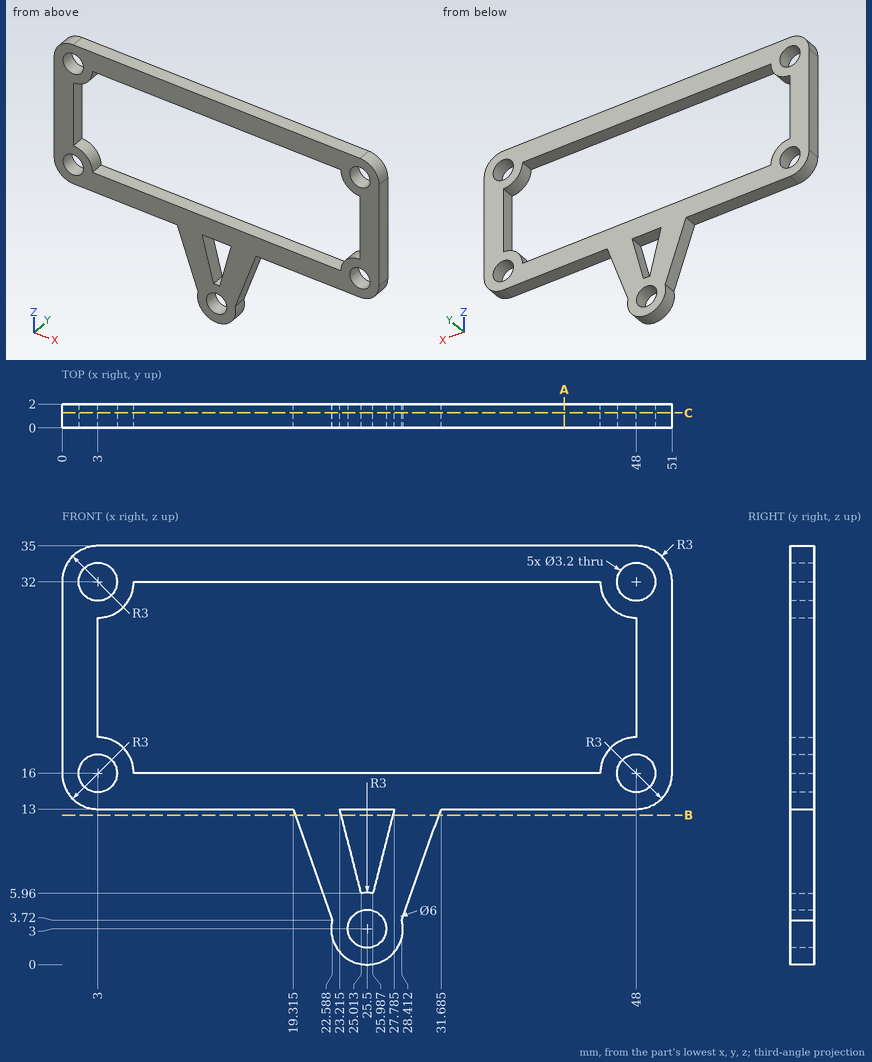
Geometry check sheet. Reference: drawing and pictorial views, mm from the part's lowest x, y, z. Coordinates: 2 decimals unless noted, no trailing zeros. Order: outer loops, then holes, each group sorted by start corner. A loop starts at its lowest first (then second) coordinate and runs counter-clockwise, first axis right, second up. Notation, with made-up numbers: (-18.5, 43.5) -> (10.5, 43.5) arc R16 ccw to (10.5, 70.5) -> close; hole circle Ø3 at (22, -31.5). An arc over 180 degrees is marked (long way). Use CSV: the item, a comma, the result in double quotes. Start each with the question number.
Q1. Depth check by flat-ended pin: P1, Ø1, axis at x = 24.5, y = 0.5, coming from the -Z side; P2, Ø1, axis at x = 40.5, y = 2, coming from the -Z side. Enter the tip coordinate at first touch or a pass-through.
Q2. Section check C-C, the plane y = 1.25. Give the number of separate pieces and of enclosed holes in the cut face.
Q3. Thickness scan on line 1 along Z through (x, y) = (34.5, 0.2); line 2 along X through (y, z) = (0.25, 20); line 3 along X through (y, z) = (0.2, 31). Record the ranges inside material, lowest first.
Q4. Section check B-B, the plane z = 12.5. Record the cut outline in (x, y).
Q5. Section check A-A, the plane x = 42. Record the cut outline in (y, z).
Returned:
1,P1,"stops at z = 0.04"
1,P2,"stops at z = 13"
2,separate pieces,"1"
2,enclosed holes,"7"
3,line 1,"z = 13 to 16, 32 to 35"
3,line 2,"x = 0 to 3, 48 to 51"
3,line 3,"x = 0 to 1.75, 4.25 to 5.83, 45.17 to 46.75, 49.25 to 51"
4,outline,"(19.49, 0) -> (23.34, 0) -> (23.34, 2) -> (19.49, 2) -> close; (27.66, 0) -> (31.51, 0) -> (31.51, 2) -> (27.66, 2) -> close"
5,outline,"(0, 13) -> (2, 13) -> (2, 16) -> (0, 16) -> close; (0, 32) -> (2, 32) -> (2, 35) -> (0, 35) -> close"
